Autodesk Inventor part; units mm, degrees
ref_plane "YZ Plane" through (0, 0, 0) normal (1, 0, 0) x (0, 1, 0)
ref_plane "XZ Plane" through (0, 0, 0) normal (0, 1, 0) x (-1, 0, 0)
ref_plane "XY Plane" through (0, 0, 0) normal (0, 0, 1) x (1, 0, 0)
sketch "スケッチ1" plane through (0, 0, 0) normal (0, 0, 1) x (1, 0, 0)
  circle A0 centre (0, 0) radius 4
  dimension "d13" = 8
extrude "押し出し1" add sketch "スケッチ1" along normal mid plane 30
sketch "スケッチ2" plane through (0, 0, 15) normal (0, 0, 1) x (1, 0, 0)
  point P0 (0, 0)
  point P1 (0, 0)
hole "穴1" at (0, 0, 15) direction (0, 0, -1) diameter 3.242 depth 11.8 tip angle 118
mirror "ミラー1" about plane through (0, 0, 0) normal (0, 0, 1) of "穴1"
chamfer "面取り1" distance 0.2 angle 45 4 edges at (0, 1.621, 15) (-4, 0, 15) (-4, 0, -15) (0, 1.621, -15)
properties part number "unir-spacer2" material "鋼、炭素鋼"
Work out the finished part from the listing and answer in its coordinate system (mm). A direction names the side the tool comes from. Coordinates: 2 decimals unless noted, no trailing zeros. Loops run counter-clockwise (first coordinate to the right, second up) from the corner with the lowest first, then second, coordinate; pieces in that order, holes last. Notation, with made-up numbers: (16, -13.5) -> (44, -13.5) arc R23 ccw to (44, -4.5) -> close; hole circle Ø8 at (-30.75, 0). An arc over 180 degrees is marked (long way). Write each question's results on one line, items separated by ' | '. Start each with the question number.
1) Consider line 1 along Y through (x, z) = (0, 8.75); line 2 along X through (y, z) = (-0.75, -12); line 3 along Y through (x, z) = (-1.25, -10.5). Determine where each line is inside the solid, lowest interval first.
2) For faces 1 (the cylindrical face through (-1.438, -0.748, -8.919)), 2 (the conical face through (-0.275, 0.061, 2.395)), determine the directions among +Z, -Z, +X, -X, +Y, -Y from which every point of the face is accessible in a straight line to the end or side of a thin tool.
3) The mould has two halves that part along X. Classify faces 3 (the cylindrical face through (1.438, -0.748, 8.919)), 4 (the flat face through (2, 1, 15)), 5 (the cylindrical face through (-0.867, 3.905, -0.207)): pulls with the +X half, pulls with the -X half, needs draft (parallel to the pull), parting line crosses it, or undercut.
4) Find section A-A on z = 12.5. Determine the outline of the cut face in (x, y).
5) Flat-ended cylindrical pins translate along their axes: P1, Ø2.5, axis at x = 0, y = 0, coming from the +Z side; P2, Ø1.5, axis at x = -1, z = 12, coming from the +Y side; P3, Ø3, axis at x = 2, z = 8, coming from the -Y side. Find the tip coordinate at first contact, or state that the pin passes through.
Response values:
1) line 1: y = -4 to -1.62, 1.62 to 4 | line 2: x = -3.93 to -1.44, 1.44 to 3.93 | line 3: y = -3.8 to -1.03, 1.03 to 3.8
2) face 1: -Z | face 2: +Z
3) face 3: undercut | face 4: needs draft | face 5: parting line crosses it
4) outline: circle Ø8 at (0, 0); hole circle Ø3.24 at (0, 0)
5) P1: stops at z = 2.98 | P2: stops at y = 3.99 | P3: stops at y = -3.97
